Autodesk Inventor part; units mm, degrees
ref_plane "YZ Plane" through (0, 0, 0) normal (1, 0, 0) x (0, 1, 0)
ref_plane "XZ Plane" through (0, 0, 0) normal (0, 1, 0) x (-1, 0, 0)
ref_plane "XY Plane" through (0, 0, 0) normal (0, 0, 1) x (1, 0, 0)
sketch "Base" plane through (0, 0, 0) normal (0, 0, 1) x (1, 0, 0)
  circle A0 centre (0, 7.375) radius 56.125 construction
  line L0 (0, -79.425) -> (0, 94.175) construction
  circle A1 centre (0, 7.375) radius 62
  line L1 (-34.5, -17.2623) -> (-48.798, -11.1931) construction
  point P0 (0, 0)
  point P1 (0, -28.5)
  dimension "d1" = 124
  dimension "d39" = 5.875
extrude "Plate1" add sketch "Base" along normal blind 5
sketch "HubCenterHole" plane through (0, 7.375, 5) normal (0, 0, 1) x (1, 0, 0)
  circle A0 centre (0, 0) radius 15 construction
  circle A1 centre (0, 0) radius 15.25
  point P0 (0, -7.375)
  dimension "d79" = 0.25
extrude "HubCenterHoleFeature" cut sketch "HubCenterHole" against normal blind 5
sketch "HubMountHoles" plane through (0, 7.375, 5) normal (0, 0, 1) x (1, 0, 0)
  circle A0 centre (0, -23.75) radius 2.5 construction
  circle A1 centre (-20.5681, -11.875) radius 2.5 construction
  circle A2 centre (-20.5681, 11.875) radius 2.5 construction
  circle A3 centre (0, 23.75) radius 2.5 construction
  circle A4 centre (20.5681, 11.875) radius 2.5 construction
  circle A5 centre (20.5681, -11.875) radius 2.5 construction
  circle A6 centre (0, -23.75) radius 2.5 construction
  circle A7 centre (0, -23.75) radius 2.2
  circle A8 centre (20.5681, -11.875) radius 2.2
  circle A9 centre (20.5681, 11.875) radius 2.2
  circle A10 centre (0, 23.75) radius 2.2
  circle A11 centre (-20.5681, -11.875) radius 2.2
  circle A12 centre (-20.5681, 11.875) radius 2.2
  point P0 (0, -7.375)
extrude "HubMountHolesFeature" cut sketch "HubMountHoles" against normal blind 5
sketch "BracketMountHoles" plane through (0, 7.375, 5) normal (0, 0, 1) x (1, 0, 0)
  circle A0 centre (-35, -19.4802) radius 2 construction
  circle A1 centre (35, -19.4802) radius 2 construction
  circle A2 centre (-35, 22.9931) radius 2 construction
  circle A3 centre (-35, -19.4802) radius 2 construction
  arc A4 (-56, -19.7436) -> (-50, -25.7436) centre (-50, -19.7436) ccw construction
  line L0 (-22, -25.7436) -> (-50, -25.7436) construction
  line L1 (-22, -25.7436) -> (-22, 29.2564) construction
  line L2 (-50, 29.2564) -> (-22, 29.2564) construction
  arc A5 (-50, 29.2564) -> (-56, 23.2564) centre (-50, 23.2564) ccw construction
  line L3 (-56, -19.7436) -> (-56, 23.2564) construction
  circle A6 centre (35, 22.9931) radius 2 construction
  circle A7 centre (35, -19.4802) radius 2 construction
  arc A8 (50, -25.7436) -> (56, -19.7436) centre (50, -19.7436) ccw construction
  line L4 (56, -19.7436) -> (56, 23.2564) construction
  arc A9 (56, 23.2564) -> (50, 29.2564) centre (50, 23.2564) ccw construction
  line L5 (50, 29.2564) -> (22, 29.2564) construction
  line L6 (22, -25.7436) -> (22, 29.2564) construction
  line L7 (22, -25.7436) -> (50, -25.7436) construction
  circle A10 centre (-35, -19.4802) radius 1.7
  circle A11 centre (-35, 22.9931) radius 1.7
  circle A12 centre (35, -19.4802) radius 1.7
  circle A13 centre (35, 22.9931) radius 1.7
  point P0 (0, -7.375)
  dimension "d88" = 4
  dimension "d89" = 3.4
  dimension "d90" = 3.4
  dimension "d91" = 3.4
  dimension "d92" = 3.4
extrude "BracketMountHolesFeature" cut sketch "BracketMountHoles" against normal blind 5
equation "\"d12\" = Thickness"
equation "\"BendRadius\" = Thickness"
equation "\"BendReliefWidth\" = Thickness"
equation "\"BendReliefDepth\" = 0.5 * Thickness"
equation "\"TransitionRadius\" = BendRadius"
equation "\"JacobiRadiusSize\" = BendRadius"
equation "\"GapSize\" = Thickness"
properties part number "NeckBase"
The listing builds one solid part. Answer for the finished solid, in the listing's coordinates (mm). Give positions to 0.01 mm unless a question says otherwise; leave off trailing zeros. Write each loop counter-clockwise with the first axis right and the second up, starting at its lowest first coordinate (ties: lowest second). Pieces come first, ordered by that corner, then holes. Notation, with made-up numbers: (-18, -24.5) -> (40, -24.5) arc R19 ccw to (40, -5.5) -> close; hole circle Ø4 at (-19, -5.5). An arc over 180 degrees is marked (long way). Use one line per item in the form item = value.
1) Section C-C on z = 3.95 is taken. Count the separate pieces of the cut face and the enclosed holes in it, plus the area to 3 significant figures.
Result:
separate_pieces = 1
enclosed_holes = 11
area = 11,200 mm²
2) Straight lines are drawn through the part: probe 1 along Y at (x, z) = (36.5, 3.4); probe 2 along Y at (x, z) = (35, 2.25); probe 3 along X at (y, z) = (8.5, 2.75). For each, find the intervals that lie inside material, in ascending order.
Result:
probe_1 = -42.74 to -12.91, -11.31 to 29.57, 31.17 to 57.49
probe_2 = -43.8 to -13.81, -10.41 to 28.67, 32.07 to 58.55
probe_3 = -61.99 to -15.21, 15.21 to 61.99
3) Each of these flat-tipped pins is pushed along its axis until it touches: P1, Ø4.5, axis at x = -35, y = 30.37, coming from the -Z side; P2, Ø1, axis at y = -42, z = 1.5, coming from the -X side; P3, Ø3.5, axis at x = 20.57, y = 19.25, coming from the -Z side; P4, Ø2, axis at y = 24.5, z = 3, coming from the +X side. Where does it stop, or does it pass through?
Result:
P1 = 0
P2 = -38.15
P3 = through
P4 = 59.87
4) Section B-B on x = -20 is taken. Write down the section's boundary in (y, z), plus the area to 3 significant figures.
Result:
outline = (-51.31, 0) -> (-6.63, 0) -> (-6.63, 5) -> (-51.31, 5) -> close; (-2.37, 0) -> (17.12, 0) -> (17.12, 5) -> (-2.37, 5) -> close; (21.38, 0) -> (66.06, 0) -> (66.06, 5) -> (21.38, 5) -> close
area = 544 mm²
5) Section A-A on x = 0 is taken. Write down the section's boundary in (y, z) (3 decimals).
Result:
outline = (-54.625, 0) -> (-18.575, 0) -> (-18.575, 5) -> (-54.625, 5) -> close; (-14.175, 0) -> (-7.875, 0) -> (-7.875, 5) -> (-14.175, 5) -> close; (22.625, 0) -> (28.925, 0) -> (28.925, 5) -> (22.625, 5) -> close; (33.325, 0) -> (69.375, 0) -> (69.375, 5) -> (33.325, 5) -> close
6) For a pull along Y with two mould halves and no side action, classify faces 1 (the cylindrical face through (-8.071, -54.097, 2.465)), 2 (the cylindrical face through (18.95, -3.01, 2.54)), 3 (the flat face through (13, -6, 0)) as +Y half, -Y half, draft (parallel to the pull), parting line (faces both ways), or undercut.
Result:
face_1 = parting line
face_2 = undercut
face_3 = draft
7) Section D-D on y = -32 is taken. Write down the section's boundary in (x, z), plus the area to 3 significant figures.
Result:
outline = (-47.89, 0) -> (47.89, 0) -> (47.89, 5) -> (-47.89, 5) -> close
area = 479 mm²
